Geometry: see drawing. Coordinates: mm, zero at the bounding-box minimum. Round coordinates to 2 decimals unless told otherwise and drop trailing zeros. Order: outer loops, then holes, each group sorted by start corner. A loop starts at its lowest first (then second) coordinate and runs counter-clockwise, first axis right, second up. Notation, with made-up numbers: (9, 25) -> (50, 25) arc R30 cw to (50, 53) -> close; hole circle Ø2 at (34, 64.5). An arc over 180 degrees is marked (long way). Use a Markdown table: item, result.
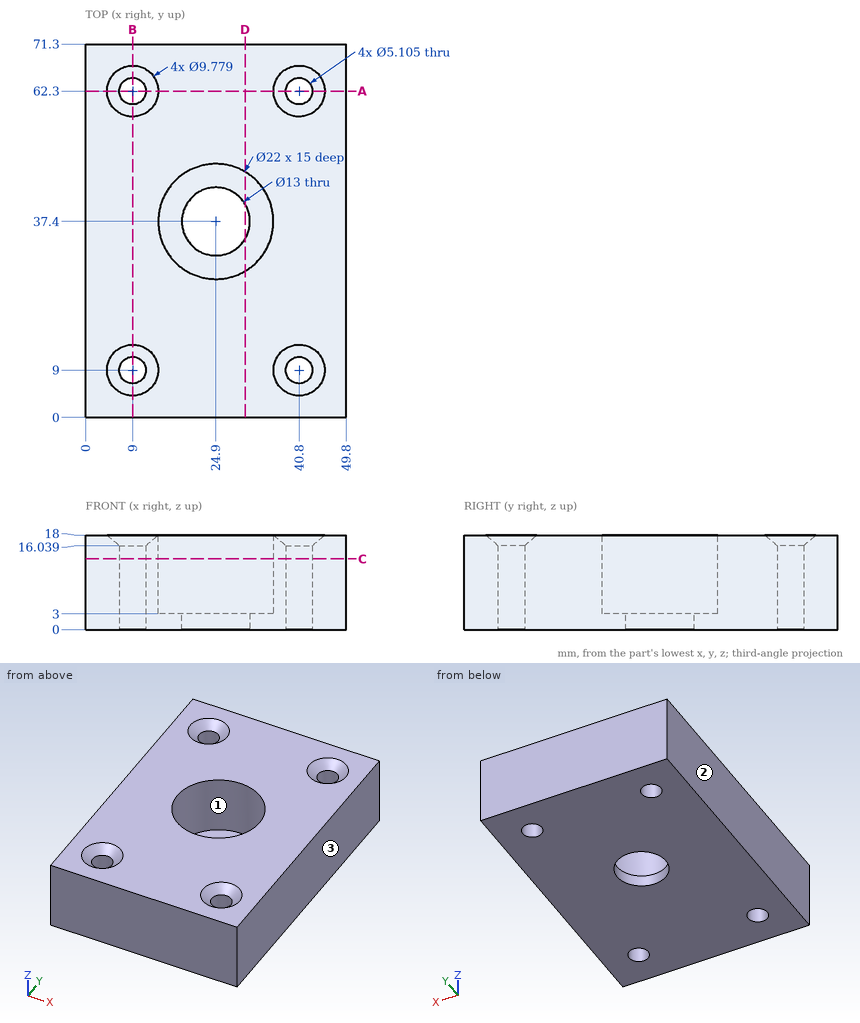
1) Ray query, probe 1 along X at (y, z) = (9, 8.5); probe 2 along Y at (x, z) = (9, 11); probe 3 along Y at (x, z) = (24.9, 6.25). Return the intervals inside material, ascending.
Answer key:
| item | result |
|---|---|
| probe 1 | x = 0 to 6.45, 11.55 to 38.25, 43.35 to 49.8 |
| probe 2 | y = 0 to 6.45, 11.55 to 59.75, 64.85 to 71.3 |
| probe 3 | y = 0 to 26.4, 48.4 to 71.3 |
2) Cut plane A-A on y = 62.3. Return loops of the section in (x, z).
Answer key:
| item | result |
|---|---|
| outline | (0, 0) -> (6.45, 0) -> (6.45, 16.04) -> (4.11, 18) -> (0, 18) -> close; (11.55, 0) -> (38.25, 0) -> (38.25, 16.04) -> (35.91, 18) -> (13.89, 18) -> (11.55, 16.04) -> close; (43.35, 0) -> (49.8, 0) -> (49.8, 18) -> (45.69, 18) -> (43.35, 16.04) -> close |
3) Cut plane D-D on x = 30.5. Return loops of the section in (y, z).
Answer key:
| item | result |
|---|---|
| outline | (0, 0) -> (34.1, 0) -> (34.1, 3) -> (27.93, 3) -> (27.93, 18) -> (0, 18) -> close; (40.7, 0) -> (71.3, 0) -> (71.3, 18) -> (46.87, 18) -> (46.87, 3) -> (40.7, 3) -> close |
4) Draft query along X for the marked faces 1, 2 and 3. Return one class per face: released by +X, released by -X, zero draft, split by the parting line, or undercut.
Answer key:
| item | result |
|---|---|
| face 1 | undercut |
| face 2 | released by -X |
| face 3 | released by +X |
5) Cut plane C-C on z = 13.5. Return loops of the section in (x, y) (1 decimal).
Answer key:
| item | result |
|---|---|
| outline | (0, 0) -> (49.8, 0) -> (49.8, 71.3) -> (0, 71.3) -> close; hole circle Ø5.1 at (9, 9); hole circle Ø5.1 at (9, 62.3); hole circle Ø22 at (24.9, 37.4); hole circle Ø5.1 at (40.8, 9); hole circle Ø5.1 at (40.8, 62.3) |
6) Contact query for a flat-ended pin moving along its axis: P1, Ø8, axis at x = 9, y = 62.3, coming from the +Z side (1 decimal). Output: stop coordinate, or through.
Answer key:
| item | result |
|---|---|
| P1 | stops at z = 17.3 |
7) Cut plane B-B on x = 9. Return loops of the section in (y, z).
Answer key:
| item | result |
|---|---|
| outline | (0, 0) -> (6.45, 0) -> (6.45, 16.04) -> (4.11, 18) -> (0, 18) -> close; (11.55, 0) -> (59.75, 0) -> (59.75, 16.04) -> (57.41, 18) -> (13.89, 18) -> (11.55, 16.04) -> close; (64.85, 0) -> (71.3, 0) -> (71.3, 18) -> (67.19, 18) -> (64.85, 16.04) -> close |
